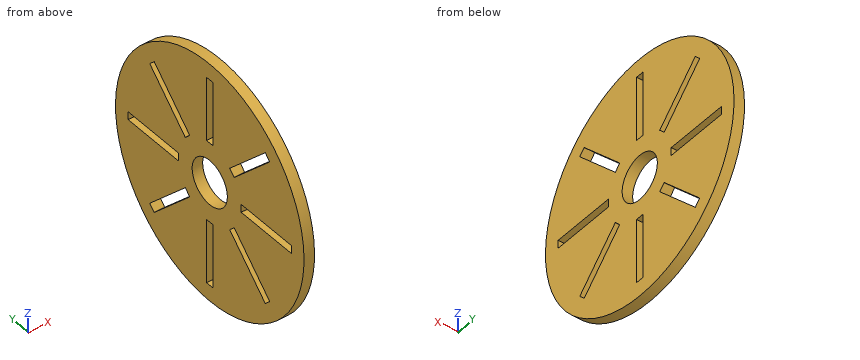
from build123d import *

# Parameters (mm, degrees)
SKETCH1_R           = 15
BOSS_EXTRUDE1_DEPTH = 1.3
SKETCH2_R           = 2.8
CUT_EXTRUDE1_DEPTH  = 22.252999788
SKETCH3_W           = 1
SKETCH3_H           = 8
SKETCH3_W_2         = 8
SKETCH3_H_2         = 1
CUT_EXTRUDE2_DEPTH  = 22.252999788


with BuildPart() as part:
    # Sketch1 → Boss-Extrude1 (new body)
    with BuildSketch(Plane(origin=(0, 0, 0), x_dir=(0, 0, -1), z_dir=(1, 0, 0))):
        Circle(SKETCH1_R)
    extrude(amount=BOSS_EXTRUDE1_DEPTH)

    # Sketch2 → Cut-Extrude1 (cut, through all)
    with BuildSketch(Plane(origin=(1.3, 0, 0), x_dir=(0, 0, -1), z_dir=(1, 0, 0))):
        Circle(SKETCH2_R)
    extrude(amount=-CUT_EXTRUDE1_DEPTH, mode=Mode.SUBTRACT)

    # Sketch3 → Cut-Extrude2 (cut, through all)
    with BuildSketch(Plane(origin=(1.3, 0, 0), x_dir=(0, 0, -1), z_dir=(1, 0, 0))):
        Polygon((-8.838834765, -9.545941546), (-3.181980515, -3.889087297), (-3.889087297, -3.181980515), (-9.545941546, -8.838834765), align=None)
        Polygon((9.545941546, -8.838834765), (3.889087297, -3.181980515), (3.181980515, -3.889087297), (8.838834765, -9.545941546), align=None)
        Polygon((-9.545941546, 8.838834765), (-3.889087297, 3.181980515), (-3.181980515, 3.889087297), (-8.838834765, 9.545941546), align=None)
        Polygon((9.545941546, 8.838834765), (3.889087297, 3.181980515), (3.181980515, 3.889087297), (8.838834765, 9.545941546), align=None)
        with Locations((0, 9)):
            Rectangle(SKETCH3_W, SKETCH3_H)
        with Locations((9, 0)):
            Rectangle(SKETCH3_W_2, SKETCH3_H_2)
        with Locations((0, -9)):
            Rectangle(SKETCH3_W, SKETCH3_H)
        with Locations((-9, 0)):
            Rectangle(SKETCH3_W_2, SKETCH3_H_2)
    extrude(amount=-CUT_EXTRUDE2_DEPTH, mode=Mode.SUBTRACT)


solid = part.part
Check sheet for the modelled part. Datum: model origin and axes. Units: mm. Round coordinates to 2 decimals unless told otherwise and drop trailing zeros. Loops run counter-clockwise (first coordinate to the right, second up) from the corner with the lowest first, then second, coordinate; pieces in that order, holes last. Notation, with made-up numbers: (-28.5, 81.25) -> (23.5, 81.25) arc R17 ccw to (23.5, 113.25) -> close; hole circle Ø4 at (27.25, 70.25). An arc over 180 degrees is marked (long way). Put each result on its own line as item: value. Start each with the question number.
1. Section check A-A (z = 0). Enter the section's corners in (x, y).
2. Section check D-D (y = 4.25). Enter the section's corners in (x, z), plus the area to 3 significant figures.
3. Gauge pin test, flat end, axial feed: pin 1 (0.6 mm diameter, centred on x = 0.5, y = -8, fed in from -Z). Record the tip position at first contact, or that the pin passes through.
4. Section check C-C (x = 0.45). Give the number of separate pieces and of enclosed holes in the cut face, plus the area to 3 significant figures.
5. Scan lines: probe 1 along Y at (x, z) = (1.05, 0); probe 2 along Y at (x, z) = (1.2, -7.75); probe 3 along Z at (x, y) = (0.6, 4.5). Record each from-to range of solid material in increasing order.
Findings:
1. outline: (0, -15) -> (1.3, -15) -> (1.3, -13) -> (0, -13) -> close; (0, -5) -> (1.3, -5) -> (1.3, -2.8) -> (0, -2.8) -> close; (0, 2.8) -> (1.3, 2.8) -> (1.3, 5) -> (0, 5) -> close; (0, 13) -> (1.3, 13) -> (1.3, 15) -> (0, 15) -> close
2. outline: (0, -14.39) -> (1.3, -14.39) -> (1.3, -4.96) -> (0, -4.96) -> close; (0, -3.54) -> (1.3, -3.54) -> (1.3, 3.54) -> (0, 3.54) -> close; (0, 4.96) -> (1.3, 4.96) -> (1.3, 14.39) -> (0, 14.39) -> close
2. area: 33.7 mm^2
3. pin 1: stops at z = -12.87
4. separate pieces: 1
4. enclosed holes: 9
4. area: 618 mm^2
5. probe 1: y = -15 to -13, -5 to -2.8, 2.8 to 5, 13 to 15
5. probe 2: y = -12.84 to -8.46, -7.04 to -0.5, 0.5 to 7.04, 8.46 to 12.84
5. probe 3: z = -14.31 to -5.21, -3.79 to 3.79, 5.21 to 14.31
